Geometry check sheet. Reference: drawing and pictorial views, mm from the part's lowest x, y, z. A direction names the side the tool comes from. Round coordinates to 2 decimals unless told otherwise and drop trailing zeros. Write each loop counter-clockwise with the first axis right and the second up, starting at its lowest first coordinate (ties: lowest second). Pieces come first, ordered by that corner, then holes. Notation, with made-up numbers: M 25.25,-5.75 L 49.25,-5.75 A13 cw 49.25,8.25 Z; hole C 57.25,5.25 d10. An arc over 180 degrees is marked long. Answer in a Markdown table with one row per item. Add a question column.
1. Set-up check for the marked faces 1 and 2: record each of +Z, -Z, +X, -X, +Y, -Y from which the full face is reachable in a straight line by a thin tool's end or side.
2. Draft check along Y on the marked faces 3, 4, 5 and 6. Enter one of: pulls with the +Y half, pulls with the -Y half, needs draft (parallel to the pull), parting line crosses it, or undercut.
3. Sectioned sample at A-A on x = 4.5. Record the cut outline in (y, z), plus the area to 3 significant figures.
4. Go/stop test with flat-tipped pins: pin 1 Ø1 at (x, y) = (9.5, 11) entering from -Z; pin 2 Ø6.5 at (x, y) = (9.5, 3.5) entering from +Z; pin 3 Ø2 at (y, z) = (4.5, 5.5) entering from +X; pin 4 Ø4 at (y, z) = (10.5, 15) entering from -X. Record where each tip stops, or that it passes through.
5. Material ranges on probe 1 along Y at (x, z) = (4.5, 1.35); probe 2 along Y at (x, z) = (16.25, 12); probe 3 along Z at (x, y) = (12.25, 11.5), recorded low to high.
6. Sectioned sample at C-C on x = 16.25. Record the cut outline in (y, z).
7. Sectioned sample at B-B on y = 6.5. Record the cut outline in (x, z).
8. Sectioned sample at D-D on z = 12. Record the cut outline in (x, y).
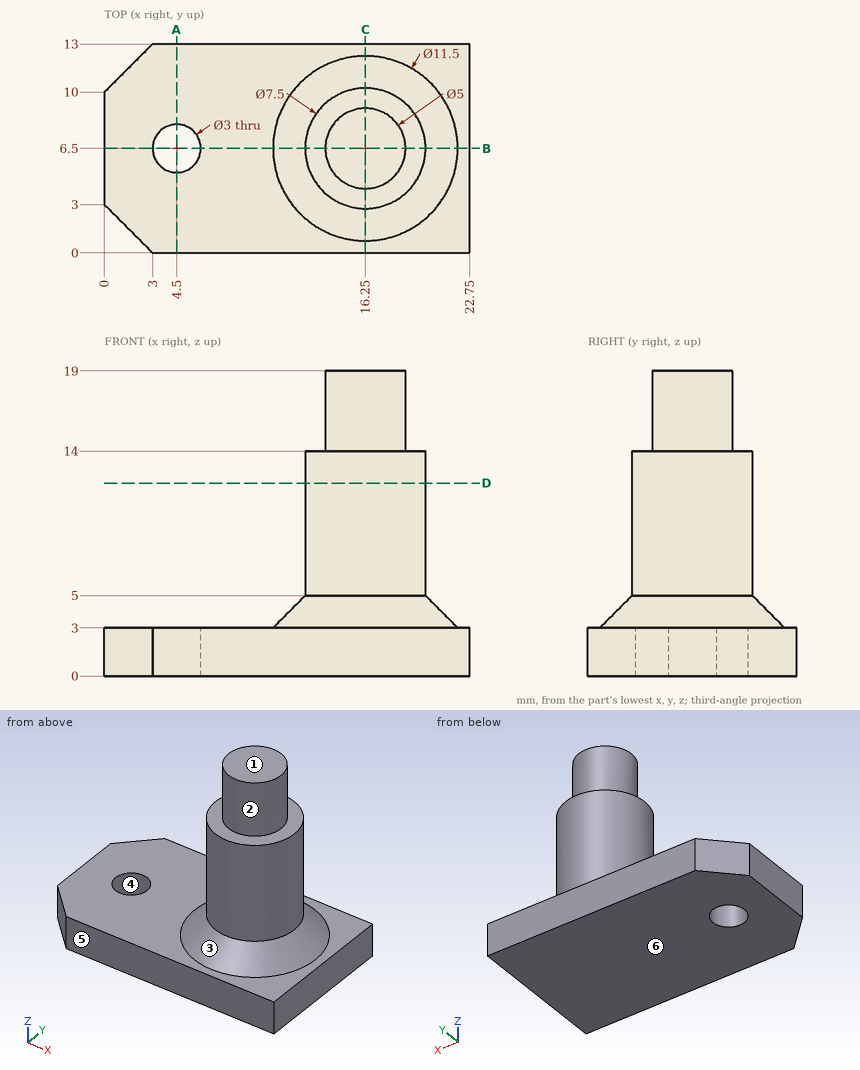
Geometry check:
| question | item | result |
|---|---|---|
| 1 | face 1 | +Z, +X, -X, +Y, -Y |
| 1 | face 2 | +Z |
| 2 | face 3 | parting line crosses it |
| 2 | face 4 | undercut |
| 2 | face 5 | pulls with the -Y half |
| 2 | face 6 | needs draft |
| 3 | outline | M 0,0 L 5,0 L 5,3 L 0,3 Z; M 8,0 L 13,0 L 13,3 L 8,3 Z |
| 3 | area | 30.0 mm2 |
| 4 | pin 1 | stops at z = 0 |
| 4 | pin 2 | stops at z = 4.61 |
| 4 | pin 3 | stops at x = 20.1 |
| 4 | pin 4 | stops at x = 13.26 |
| 5 | probe 1 | y = 0 to 5, 8 to 13 |
| 5 | probe 2 | y = 2.75 to 10.25 |
| 5 | probe 3 | z = 0 to 3 |
| 6 | outline | M 0,0 L 13,0 L 13,3 L 12.25,3 L 10.25,5 L 10.25,14 L 9,14 L 9,19 L 4,19 L 4,14 L 2.75,14 L 2.75,5 L 0.75,3 L 0,3 Z |
| 7 | outline | M 0,0 L 3,0 L 3,3 L 0,3 Z; M 6,0 L 22.75,0 L 22.75,3 L 22,3 L 20,5 L 20,14 L 18.75,14 L 18.75,19 L 13.75,19 L 13.75,14 L 12.5,14 L 12.5,5 L 10.5,3 L 6,3 Z |
| 8 | outline | C 16.25,6.5 d7.5 |
